Geometry: final body of the model. Coordinates: model frame, mm. A direction names the side the tool comes from. Give positions to 0.01 mm unless a question says otherwise; leave off trailing zeros. Loops run counter-clockwise (first coordinate to the right, second up) from the corner with the lowest first, then second, coordinate; pieces in that order, holes last. Notation, with made-up numbers: M -25.75,-32 L -15.75,-32 A24 ccw -15.75,4 Z; hole C 57.25,-15 d11. An arc over 180 degrees is marked long. Put each result on its own line as item: value.
```python
from build123d import *

# Parameters (mm, degrees)
EXTRUDE_THIN1_DEPTH      = 8
EXTRUDE_THIN1_DEPTH_BACK = 55
REVOLVE1_ANGLE           = 180
CUT_EXTRUDE1_DEPTH       = 1
CUT_EXTRUDE1_DEPTH_BACK  = 73.5
REVOLVE2_ANGLE           = 180
CUT_EXTRUDE2_DEPTH       = 1.0000001
CUT_EXTRUDE2_DEPTH_BACK  = 20.0000001


with BuildPart() as part:
    # Sketch1 → Extrude-Thin1 (new body, two sides)
    with BuildSketch(Plane.XY) as extrude_thin1_sk:
        with BuildLine():
            Line((-10.608745061, -19.461766721), (-10.608745061, 18.038233279))
            ThreePointArc((-10.608745061, 18.038233279), (-1.108745061, 27.538233279), (8.391254939, 18.038233279))
            Line((8.391254939, 18.038233279), (8.391254939, -19.461766721))
            ThreePointArc((8.391254939, -19.461766721), (-1.108745061, -28.961766721), (-10.608745061, -19.461766721))
        make_face()
        with BuildLine():
            Line((-8.608745061, -19.461766721), (-8.608745061, 18.038233279))
            ThreePointArc((-8.608745061, 18.038233279), (-1.108745061, 25.538233279), (6.391254939, 18.038233279))
            Line((6.391254939, 18.038233279), (6.391254939, -19.461766721))
            ThreePointArc((6.391254939, -19.461766721), (-1.108745061, -26.961766721), (-8.608745061, -19.461766721))
        make_face(mode=Mode.SUBTRACT)
    extrude(amount=EXTRUDE_THIN1_DEPTH)
    extrude(extrude_thin1_sk.sketch, amount=-EXTRUDE_THIN1_DEPTH_BACK)

    # Sketch3 → Revolve1 (revolve)
    with BuildSketch(Plane.XY.offset(8)):
        with BuildLine():
            Line((6.391254939, -19.461766721), (6.391254939, 18.038233279))
            ThreePointArc((6.391254939, 18.038233279), (4.194555798, 23.341534137), (-1.108745061, 25.538233279))
            Line((-1.108745061, 25.538233279), (-1.108745061, 27.538233279))
            ThreePointArc((-1.108745061, 27.538233279), (5.608769361, 24.7557477), (8.391254939, 18.038233279))
            Line((8.391254939, 18.038233279), (8.391254939, -19.461766721))
            ThreePointArc((8.391254939, -19.461766721), (5.608769361, -26.179281143), (-1.108745061, -28.961766721))
            Line((-1.108745061, -28.961766721), (-1.108745061, -26.961766721))
            ThreePointArc((-1.108745061, -26.961766721), (4.194555798, -24.76506758), (6.391254939, -19.461766721))
        make_face()
    revolve(axis=Axis((-1.108745061, 27.538233279, 8), (0, -1, 0)), revolution_arc=REVOLVE1_ANGLE)

    # Sketch4 → Cut-Extrude1 (cut, two sides)
    with BuildSketch(Plane(origin=(-1.108745061, -19.461766721, 17.5), x_dir=(1, 0, 0), z_dir=(0, 0, 1))) as cut_extrude1_sk:
        with BuildLine():
            Line((7.413248602, 27.101186929), (7.328248101, 20.145490054))
            ThreePointArc((7.328248101, 20.145490054), (5.359735954, 18.224508573), (3.438754472, 20.19302072))
            Line((3.438754472, 20.19302072), (3.523754973, 27.148717596))
            ThreePointArc((3.523754973, 27.148717596), (5.492267121, 29.069699077), (7.413248602, 27.101186929))
        make_face()
    extrude(amount=CUT_EXTRUDE1_DEPTH, mode=Mode.SUBTRACT)
    extrude(cut_extrude1_sk.sketch, amount=-CUT_EXTRUDE1_DEPTH_BACK, mode=Mode.SUBTRACT)

    # Sketch5 → Revolve2 (revolve)
    with BuildSketch(Plane(origin=(0, 0, -55), x_dir=(-1, 0, 0), z_dir=(0, 0, -1))):
        with BuildLine():
            Line((-6.391254939, -19.461766721), (-6.391254939, 18.038233279))
            ThreePointArc((-6.391254939, 18.038233279), (-4.194555798, 23.341534137), (1.108745061, 25.538233279))
            Line((1.108745061, 25.538233279), (1.108745061, 27.538233279))
            ThreePointArc((1.108745061, 27.538233279), (-5.608769361, 24.7557477), (-8.391254939, 18.038233279))
            Line((-8.391254939, 18.038233279), (-8.391254939, -19.461766721))
            ThreePointArc((-8.391254939, -19.461766721), (-5.608769361, -26.179281143), (1.108745061, -28.961766721))
            Line((1.108745061, -28.961766721), (1.108745061, -26.961766721))
            ThreePointArc((1.108745061, -26.961766721), (-4.194555798, -24.76506758), (-6.391254939, -19.461766721))
        make_face()
    revolve(axis=Axis((-1.108745061, -28.961766721, -55), (0, 1, 0)), revolution_arc=REVOLVE2_ANGLE)

    # Sketch6 → Cut-Extrude2 (cut, two sides)
    with BuildSketch(Plane(origin=(8.391254939, 0, 0), x_dir=(0, 0, -1), z_dir=(1, 0, 0))) as cut_extrude2_sk:
        Polygon((47.502612286, -35.061794905), (47.502612286, -11.65288681), (66.549267121, 7.393768025), (66.549267121, -35.061794905), align=None)
    extrude(amount=CUT_EXTRUDE2_DEPTH, mode=Mode.SUBTRACT)
    extrude(cut_extrude2_sk.sketch, amount=-CUT_EXTRUDE2_DEPTH_BACK, mode=Mode.SUBTRACT)


solid = part.part
```
Item 1: Section C-C on y = -7. Output: boundary loops of the cut face in (x, z), then the cut area to 3 significant figures.
Output values:
outline: M -10.61,-52.16 L -8.61,-52.16 L -8.61,8 A7.5 cw 6.39,8 L 6.39,-52.16 L 8.39,-52.16 L 8.39,8 A9.5 ccw -10.61,8 Z
area: 294 mm²
Item 2: Section D-D on x = 1. Output: boundary loops of the cut face in (y, z).
Output values:
outline: M -28.72,-47.5 L -26.66,-47.5 L -26.66,8 A7.2 cw -19.46,15.2 L 18.04,15.2 A7.2 cw 25.24,8 L 25.24,-55 A7.2 cw 18.04,-62.2 L 3.04,-62.2 L 5.11,-64.26 L 18.04,-64.26 A9.26 ccw 27.3,-55 L 27.3,8 A9.26 ccw 18.04,17.26 L -19.46,17.26 A9.26 ccw -28.72,8 Z
Item 3: Set-up query: faces 1 (the flat face through (6.391, 0, -23)), 2 (the cylindrical face through (-0.94, 9.56, -62.5)), 3 (the flat face through (-3, -27, -47.503)), 4 (the cylindrical face through (4.958, -1.114, 14.083)). Return all of +Z, -Z, +X, -X, +Y, -Y with unobstructed straight access to the full face (end or side cutting, diameter ignored); none if empty.
Output values:
face 1: none
face 2: -Y
face 3: -Z, +X, -X, -Y
face 4: +Z
Item 4: Section B-B on x = 5.25. Output: boundary loops of the cut face in (y, z).
Output values:
outline: M -26.52,-47.5 L -23.44,-47.5 L -23.44,8 A3.98 cw -19.46,11.98 L -0.98,11.98 L -0.98,15.06 L -19.46,15.06 A7.06 ccw -26.52,8 Z; M -0.18,-58.98 L 2.9,-62.06 L 18.04,-62.06 A7.06 ccw 25.1,-55 L 25.1,8 A7.06 ccw 18.04,15.06 L 9.39,15.06 L 9.39,11.98 L 18.04,11.98 A3.98 cw 22.02,8 L 22.02,-55 A3.98 cw 18.04,-58.98 Z
Item 5: Line query: probe 1 along X at (y, z) = (-14.5, -7); probe 2 along Y at (x, z) = (-1, -43.5); probe 3 along Z at (x, y) = (0.5, 14). Output: solid intervals per line, ascending. Write a range as [from, to].
Output values:
probe 1: [-10.61, -8.61], [6.39, 8.39]
probe 2: [-28.96, -26.96], [25.54, 27.54]
probe 3: [-64.36, -62.33], [15.33, 17.36]
Item 6: Mould query, pull axis X, two halves, no side actions, for faces 5 (the cylindrical face through (-1.274, 25.536, -23.059)), 6 (the cylindrical face through (-0.9, -0.974, 17.498)), 7 (the flat face through (5.973, -0.676, -58.48)). Classes: pulls with the +X half, pulls with the -X half, needs draft (parallel to the pull), parting line crosses it, or undercut.
Output values:
face 5: undercut
face 6: parting line crosses it
face 7: needs draft
Item 7: Section A-A on z = -11.5. Output: boundary loops of the cut face in (x, y), then the cut area to 3 significant figures.
Output values:
outline: M -10.61,-19.46 A9.5 ccw 8.39,-19.46 L 8.39,18.04 A9.5 ccw -10.61,18.04 Z; hole M -8.61,-19.46 A7.5 ccw 6.39,-19.46 L 6.39,18.04 A7.5 ccw -8.61,18.04 Z
area: 257 mm²
Item 8: Pin query (flat end, axial travel): pin 1 Ø2 at (x, z) = (0, -51) entering from -Y; pin 2 Ø1 at (y, z) = (-21, -34.5) entering from +X; pin 3 Ø1.5 at (x, y) = (0.5, 15.5) entering from -Z. Return the tip coordinate at first contact, or that it passes through.
Output values:
pin 1: y = 25.24
pin 2: x = 8.33
pin 3: z = -64.46
